Part model, mm, in its own coordinate system. Face numbers are marked on the shaded views. A direction names the side the tool comes from. Round coordinates to 2 decimals unless told otherwise and drop trailing zeros. Loops run counter-clockwise (first coordinate to the right, second up) from the corner with the lowest first, then second, coordinate; pieces in that order, holes last.
1) 3-axis set-ups, long thin cutter, end or side, ignore diameter. For the marked faces 1 and 2: which of +Z, -Z, +X, -X, +Y, -Y reach the whole face in a straight line?
2) Drop flat-ended pins along their axis: P1, Ø1.4, axis at x = 0, y = 8.5, coming from the -Z side; P2, Ø1, axis at x = 0, y = 9, coming from the +Z side; P3, Ø0.6, axis at y = 8.5, z = 0, coming from the +X side; P4, Ø1.6, axis at x = 0, z = 0, coming from the +Y side. Give the stop position or say it passes through.
3) Probe line 1 (Z direction, x = 0.1, y = 6.25); line 2 (Y direction, x = 0.7, z = 2.25); line 3 (Y direction, x = -1.95, z = 1.5). List the from-to ranges inside material, lowest first.
4) Mould opens along X. For the marked faces 3, 4 and 5 say: +X half, -X half, draft (parallel to the pull), parting line (faces both ways), or undercut.
5) Band-saw the part on A-A, the plane y = 7.5. Write the cut outline in (x, z).
from build123d import *

# Parameters (mm, degrees)
SKETCH1_RX          = 3.556
SKETCH1_RY          = 2.54
BOSS_EXTRUDE1_DEPTH = 3
SKETCH2_R           = 2.032
BOSS_EXTRUDE2_DEPTH = 6.35
SKETCH3_W           = 1.468765614
SKETCH3_H           = 1.503189808
CUT_EXTRUDE1_DEPTH  = 1.27
FILLET1_R           = 0.5


with BuildPart() as part:
    # Sketch1 → Boss-Extrude1 (new body)
    with BuildSketch(Plane(origin=(0, 0, 0), x_dir=(1, 0, 0), z_dir=(0, 1, 0))):
        with Locations(Location((0, 0), (0, 0, 109.894492076))):
            Ellipse(SKETCH1_RX, SKETCH1_RY)
    extrude(amount=BOSS_EXTRUDE1_DEPTH)

    # Sketch2 → Boss-Extrude2 (add)
    with BuildSketch(Plane(origin=(0, 3, 0), x_dir=(1, 0, 0), z_dir=(0, 1, 0))):
        with Locations(Location((0, 0, 0), (0, 0, 270))):
            Circle(SKETCH2_R)
    extrude(amount=BOSS_EXTRUDE2_DEPTH)

    # Sketch3 → Cut-Extrude1 (cut)
    with BuildSketch(Plane(origin=(0, 9.35, 0), x_dir=(1, 0, 0), z_dir=(0, 1, 0))):
        Rectangle(SKETCH3_W, SKETCH3_H)
    extrude(amount=-CUT_EXTRUDE1_DEPTH, mode=Mode.SUBTRACT)

    # Fillet1
    fillet1_edges = [part.edges().sort_by_distance(p)[0] for p in [
        (1.211452415, 0, 3.343279373),
    ]]
    fillet(fillet1_edges, radius=FILLET1_R)


solid = part.part
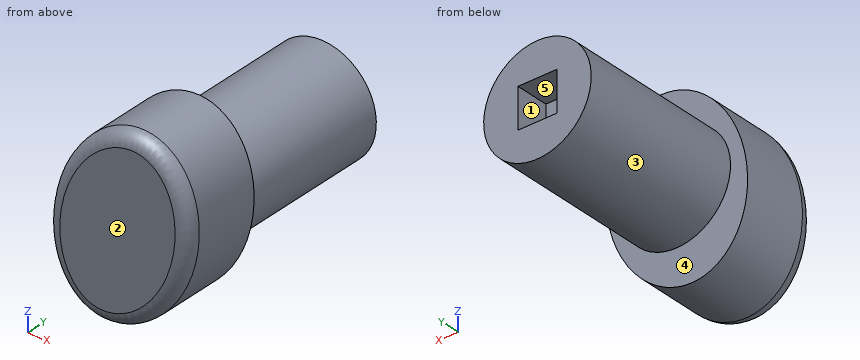
Reported:
1. face 1: +Y
1. face 2: +Z, -Z, +X, -X, -Y
2. P1: stops at z = -2.03
2. P2: stops at z = 2.03
2. P3: stops at x = 2.03
2. P4: stops at y = 9.35
3. line 1: z = -2.03 to 2.03
3. line 2: y = 0 to 3
3. line 3: y = 0.16 to 3
4. face 3: parting line
4. face 4: draft
4. face 5: undercut
5. outline: circle Ø4.06 at (0, 0)
